from build123d import *

# Parameters (mm, degrees)
SKETCH1_W             = 53
SKETCH1_H             = 34
BOSS_EXTRUDE1_DEPTH   = 5
SKETCH2_W             = 48.6
SKETCH2_H             = 31.6
CUT_EXTRUDE1_DEPTH    = 3.5
BOSS_EXTRUDE2_DEPTH   = 1
SKETCH4_W             = 1.2
SKETCH4_H             = 10
CUT_EXTRUDE2_DEPTH    = 0.5
SKETCH5_W             = 3.2
SKETCH5_H             = 30.4
CUT_EXTRUDE3_DEPTH    = 2.1
SKETCH6_W             = 5.4
SKETCH6_H             = 5.4
SKETCH6_H_2           = 4.3
BOSS_EXTRUDE3_DEPTH   = 3
SKETCH7_R             = 1.6
BOSS_EXTRUDE4_DEPTH   = 1.2
M2_TAPPED_HOLE1_D     = 1.6
M2_TAPPED_HOLE1_DEPTH = 5.2
M2_TAPPED_HOLE1_TIP   = 0.480688495


with BuildPart() as part:
    # Sketch1 → Boss-Extrude1 (new body)
    with BuildSketch(Plane(origin=(0, 0, 0), x_dir=(1, 0, 0), z_dir=(0, 1, 0))):
        with Locations((26.5, 17)):
            Rectangle(SKETCH1_W, SKETCH1_H)
    extrude(amount=BOSS_EXTRUDE1_DEPTH)

    # Sketch2 → Cut-Extrude1 (cut)
    with BuildSketch(Plane.XZ):
        with Locations((25.5, -17)):
            Rectangle(SKETCH2_W, SKETCH2_H)
    extrude(amount=-CUT_EXTRUDE1_DEPTH, mode=Mode.SUBTRACT)

    # Sketch3 → Boss-Extrude2 (add)
    with BuildSketch(Plane.XZ):
        Polygon((49.8, -1.2), (1.2, -1.2), (1.2, -12), (0.9, -12), (0.9, -0.9), (49.8, -0.9), align=None)
        Polygon((1.2, -22), (1.2, -32.8), (49.8, -32.8), (49.8, -33.1), (0.9, -33.1), (0.9, -22), align=None)
    extrude(amount=BOSS_EXTRUDE2_DEPTH)

    # Sketch4 → Cut-Extrude2 (cut)
    with BuildSketch(Plane.XZ):
        with Locations((0.6, -17)):
            Rectangle(SKETCH4_W, SKETCH4_H)
    extrude(amount=-CUT_EXTRUDE2_DEPTH, mode=Mode.SUBTRACT)

    # Sketch5 → Cut-Extrude3 (cut)
    with BuildSketch(Plane.XZ):
        with Locations((51.4, -17)):
            Rectangle(SKETCH5_W, SKETCH5_H)
    extrude(amount=-CUT_EXTRUDE3_DEPTH, mode=Mode.SUBTRACT)

    # Sketch6 → Boss-Extrude3 (add)
    with BuildSketch(Plane.XZ.offset(-3.5)):
        with Locations((3.9, -3.9)):
            Rectangle(SKETCH6_W, SKETCH6_H)
        with Locations((3.9, -30.65)):
            Rectangle(SKETCH6_W, SKETCH6_H_2)
    extrude(amount=BOSS_EXTRUDE3_DEPTH)

    # Sketch7 → Boss-Extrude4 (add)
    with BuildSketch(Plane.XZ.offset(-0.5)):
        with Locations(Location((5, -5, 0), (0, 0, 270))):
            Circle(SKETCH7_R)
        with Locations((5, -30.5)):
            Circle(SKETCH7_R)
    extrude(amount=BOSS_EXTRUDE4_DEPTH)

    # M2 Tapped Hole1
    with Locations(Plane(origin=(5, -0.7, -5), x_dir=(0, 0, -1), z_dir=(0, -1, 0))):
        with Locations((0, 0), (25.5, 0)):
            Hole(M2_TAPPED_HOLE1_D / 2, depth=M2_TAPPED_HOLE1_DEPTH)
            with Locations((0, 0, -(M2_TAPPED_HOLE1_DEPTH + M2_TAPPED_HOLE1_TIP / 2))):  # 118° drill point
                Cone(0, M2_TAPPED_HOLE1_D / 2, M2_TAPPED_HOLE1_TIP, mode=Mode.SUBTRACT)


solid = part.part
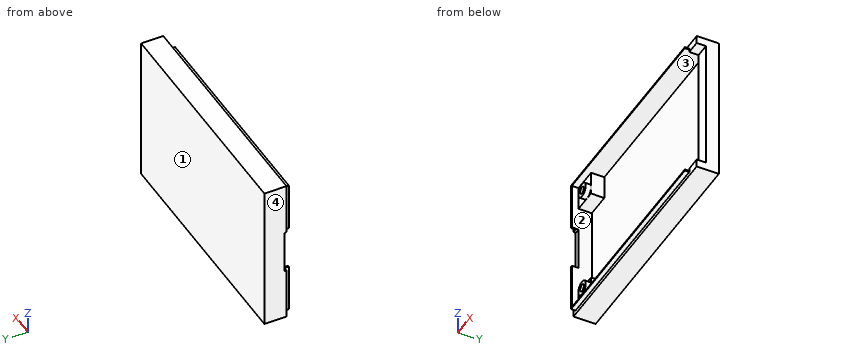
Design review of the part built by this model. Coordinates are the model's own, in mm. Face numbers are marked on the shaded views. Round coordinates to 2 decimals unless told otherwise and drop trailing zeros. Loops run counter-clockwise (first coordinate to the right, second up) from the corner with the lowest first, then second, coordinate; pieces in that order, holes last. Notation, with made-up numbers: M 60,25 L 113,25 A22 cw 113,46 Z; hole C 33,-40 d9. An arc over 180 degrees is marked long. Answer as a JSON object with one key per item and string values.
Item 1: We need section A-A on y = 1.4. Give the boundary of the cut face in (x, z), and give its area (3 significant figures).
Answer sheet:
{"outline": "M 0,-34 L 53,-34 L 53,-32.2 L 49.8,-32.2 L 49.8,-32.8 L 6.6,-32.8 L 6.6,-28.5 L 1.2,-28.5 L 1.2,-6.6 L 6.6,-6.6 L 6.6,-1.2 L 49.8,-1.2 L 49.8,-1.8 L 53,-1.8 L 53,0 L 0,0 Z; hole C 5,-30.5 d1.6; hole C 5,-5 d1.6", "area": "217 mm^2"}
Item 2: Wall thickness on L1, parallel to X at y = 0.3, z = -5; L2, parallel to Z at x = 5, y = 1.2; L3, parallel to Z at x = 7.5, y = 0.35: over which ranges is each line inside the solid? List them lowest first. Write a range as from..to.
Answer sheet:
{"L1": "x = 0..1.2, 3.4..4.2, 5.8..6.6", "L2": "z = -34..-31.3, -29.7..-28.5, -6.6..-5.8, -4.2..0", "L3": "z = -34..-32.8, -1.2..0"}
Item 3: The part is to be moulded in two halves that separate along X. For the marked faces 1, 2, 3 and 4, say which applies: pulls with the +X half, pulls with the -X half, needs draft (parallel to the pull), parting line crosses it, or undercut.
Answer sheet:
{"face 1": "needs draft", "face 2": "undercut", "face 3": "undercut", "face 4": "pulls with the -X half"}
Item 4: Clearance check with flat-ended pins moving along their axes: P1, Ø6, axis at x = 3, z = -3, coming from the -Y side; P2, Ø0.8, axis at y = -0.5, z = -8.5, coming from the -X side; P3, Ø0.8, axis at x = 16, y = -0.5, coming from the +Z side; P4, Ø3.5, axis at x = 3, z = -30, coming from the -Y side. State where each tip first meets the part, or that it passes through.
Answer sheet:
{"P1": "stops at y = -1", "P2": "stops at x = 0.9", "P3": "stops at z = -0.9", "P4": "stops at y = -0.7"}
Item 5: We need section B-B on z = -9. Give the boundary of the cut face in (x, y).
Answer sheet:
{"outline": "M 0,0 L 0.9,0 L 0.9,-1 L 1.2,-1 L 1.2,3.5 L 49.8,3.5 L 49.8,2.1 L 53,2.1 L 53,5 L 0,5 Z"}
Item 6: We need section C-C on x = 10. Give the boundary of the cut face in (y, z).
Answer sheet:
{"outline": "M -1,-33.1 L 0,-33.1 L 0,-34 L 5,-34 L 5,0 L 0,0 L 0,-0.9 L -1,-0.9 L -1,-1.2 L 3.5,-1.2 L 3.5,-32.8 L -1,-32.8 Z"}
